Here's how the part is built. I have some questions about the finished solid (model axes, mm). Coordinates: 2 decimals unless noted, no trailing zeros. Write each loop counter-clockwise with the first axis right and the second up, starting at its lowest first coordinate (ties: lowest second). Pieces come first, ordered by that corner, then holes.
Item 1: I want a section at B-B (y = 2.75). Please give me the cut outline in (x, z).
Item 2: I'm going to push flat-ended pins straight in: P1, Ø1.9, axis at y = 1.5, z = -226.5, coming from the +X side; P2, Ø1.9, axis at x = 204.5, y = 3, coming from the +Z side. Where does each tip first touch, or does it pass through?
Item 3: I want a section at C-C (z = -409.5). Please give me the cut outline in (x, y), and give its area (3 significant figures).
Item 4: I want a section at D-D (x = 257). Please give me the cut outline in (y, z).
Item 5: Please list where these lines run through material, in increasing order: line 1 (Z direction, x = 103, y = 5.5); line 2 (Z direction, x = 48.5, y = 4); line 3 (X direction, y = 6, z = -351).
Item 6: I want a section at A-A (x = 128.5). Please give me the cut outline in (y, z).
from build123d import *

# Parameters (mm, degrees)
SKETCH1_W           = 310.134
SKETCH1_H           = 469.9
BOSS_EXTRUDE1_DEPTH = 6.35
SKETCH2_W           = 254
SKETCH2_H           = 127
CUT_EXTRUDE1_DEPTH  = 564.053665698
FILLET1_R           = 38.1
SKETCH3_W           = 184.15
SKETCH3_H           = 107.95
CUT_EXTRUDE2_DEPTH  = 564.053665698


with BuildPart() as part:
    # Sketch1 → Boss-Extrude1 (new body)
    with BuildSketch(Plane(origin=(0, 0, 0), x_dir=(1, 0, 0), z_dir=(0, 1, 0))):
        with Locations((155.067, 234.95)):
            Rectangle(SKETCH1_W, SKETCH1_H)
    extrude(amount=BOSS_EXTRUDE1_DEPTH)

    # Sketch2 → Cut-Extrude1 (cut, through all)
    with BuildSketch(Plane(origin=(0, 6.35, 0), x_dir=(1, 0, 0), z_dir=(0, 1, 0))):
        with Locations((183.134, 234.95)):
            Rectangle(SKETCH2_W, SKETCH2_H)
    extrude(amount=-CUT_EXTRUDE1_DEPTH, mode=Mode.SUBTRACT)

    # Fillet1
    fillet1_edges = [part.edges().sort_by_distance(p)[0] for p in [
        (56.134, 3.175, -171.45),
        (56.134, 3.175, -298.45),
    ]]
    fillet(fillet1_edges, radius=FILLET1_R)

    # Sketch3 → Cut-Extrude2 (cut, through all)
    with BuildSketch(Plane(origin=(0, 6.35, 0), x_dir=(1, 0, 0), z_dir=(0, 1, 0))):
        with Locations((135.509, 384.175)):
            Rectangle(SKETCH3_W, SKETCH3_H)
    extrude(amount=-CUT_EXTRUDE2_DEPTH, mode=Mode.SUBTRACT)


solid = part.part
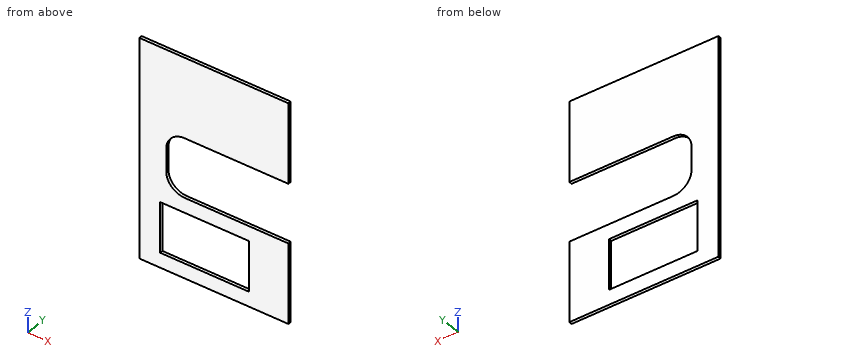
Answer:
1. outline: (0, -469.9) - (310.13, -469.9) - (310.13, -298.45) - (94.23, -298.45) arc R38.1 cw to (56.13, -260.35) - (56.13, -209.55) arc R38.1 cw to (94.23, -171.45) - (310.13, -171.45) - (310.13, 0) - (0, 0) - close; hole (43.43, -438.15) - (227.58, -438.15) - (227.58, -330.2) - (43.43, -330.2) - close
2. P1: stops at x = 56.13
2. P2: stops at z = 0
3. outline: (0, 0) - (43.43, 0) - (43.43, 6.35) - (0, 6.35) - close; (227.58, 0) - (310.13, 0) - (310.13, 6.35) - (227.58, 6.35) - close
3. area: 800 mm2
4. outline: (0, -469.9) - (6.35, -469.9) - (6.35, -298.45) - (0, -298.45) - close; (0, -171.45) - (6.35, -171.45) - (6.35, 0) - (0, 0) - close
5. line 1: z = -469.9 to -438.15, -330.2 to -298.45, -171.45 to 0
5. line 2: z = -469.9 to -438.15, -330.2 to 0
5. line 3: x = 0 to 43.43, 227.58 to 310.13
6. outline: (0, -469.9) - (6.35, -469.9) - (6.35, -438.15) - (0, -438.15) - close; (0, -330.2) - (6.35, -330.2) - (6.35, -298.45) - (0, -298.45) - close; (0, -171.45) - (6.35, -171.45) - (6.35, 0) - (0, 0) - close
